```python
from build123d import *

# Parameters (mm, degrees)
SKETCH2_W           = 50.8
SKETCH2_H           = 12.7
BOSS_EXTRUDE1_DEPTH = 88.9
FILLET2_R           = 3.175
SHELL1_T            = 6.35


with BuildPart() as part:
    # Sketch2 → Boss-Extrude1 (new body)
    with BuildSketch(Plane(origin=(0, 0, 0), x_dir=(1, 0, 0), z_dir=(0, 1, 0))):
        with Locations((25.4, 6.35)):
            Rectangle(SKETCH2_W, SKETCH2_H)
    extrude(amount=BOSS_EXTRUDE1_DEPTH)

    # Fillet2
    fillet2_edges = [part.edges().sort_by_distance(p)[0] for p in [
        (50.8, 44.45, 0),
        (0, 44.45, 0),
    ]]
    fillet(fillet2_edges, radius=FILLET2_R)

    # Shell1
    shell1_openings = [part.faces().sort_by_distance(p)[0] for p in [
        (25.4, 0, -6.38808439),
        (25.4, 88.9, -6.38808439),
        (25.4, 44.45, -12.7),
    ]]
    offset(amount=SHELL1_T, openings=shell1_openings, kind=Kind.INTERSECTION)


solid = part.part
```
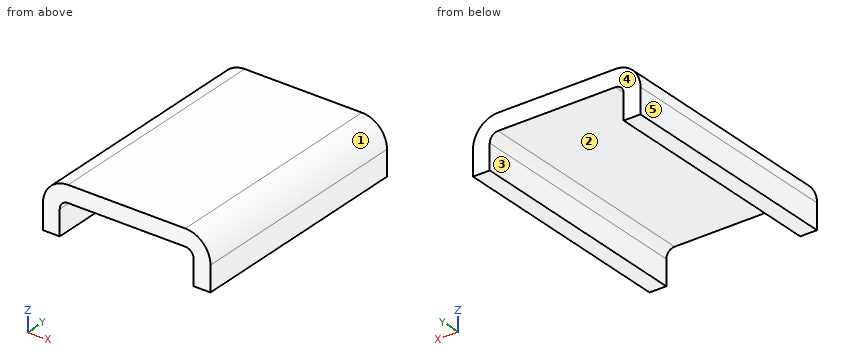
Could you check a few things on this model? Use its own coordinates, in mm. Face numbers are marked on the shaded views. A direction names the side the tool comes from. Give positions to 0.01 mm unless a question says otherwise; leave off trailing zeros. Write each loop counter-clockwise with the first axis right and the second up, starting at its lowest first coordinate (ties: lowest second). Pieces come first, ordered by that corner, then holes. Notation, with made-up numbers: (25.25, 7.25) - (77.25, 7.25) arc R23 cw to (77.25, 42.25) - close; hole circle Ø5 at (3, -15.5). An arc over 180 degrees is marked (long way). One line per item, written item: value. Start each with the question number.
Item 1: Imagine slicing it at A-A, the plane y = 62. List the corners of the cut face in (x, z) for me (3 decimals), and give its area (3 significant figures).
Item 2: Imagine slicing it at B-B, the plane z = -7.25. List the corners of the cut face in (x, y) for me.
Item 3: Imagine slicing it at C-C, the plane x = 28. List the corners of the cut face in (y, z) for me, and give its area (3 significant figures).
Item 4: I'm going to push flat-ended pins straight in: pin 1 (1.5 mm diameter, centred on y = 73, z = 3.5, fed in from +X); pin 2 (10 mm diameter, centred on y = 38.5, z = 1.5, fed in from +X); pin 3 (5 mm diameter, centred on x = 34.5, y = 69.5, fed in from -Z). Where does each tip first touch, or does it pass through?
Item 5: Which directions (+Z, -Z, +X, -X, +Y, -Y) give clear straight access to the entire face, cutting with the end or side of a thin tool? Please do the marked faces 1 and 2.
Item 6: Imagine slicing it at D-D, the plane z = 2. List the corners of the cut face in (x, y) for me.
Item 7: If we mould it in two halves opening along X, with no side actions, what happens to the marked faces 3, 4 and 5? For each: +X half, -X half, draft (parallel to the pull), parting line (faces both ways), or undercut.
Item 8: Please list where these lines run through material, in increasing order: line 1 (X direction, y = 79, z = -11.5); line 2 (Z direction, x = 25, y = 46). Write a range as from..to.
Geometry says:
1. outline: (-6.35, -12.7) - (0, -12.7) - (0, -3.175) arc R3.175 cw to (3.175, 0) - (47.625, 0) arc R3.175 cw to (50.8, -3.175) - (50.8, -12.7) - (57.15, -12.7) - (57.15, -3.175) arc R9.525 ccw to (47.625, 6.35) - (3.175, 6.35) arc R9.525 ccw to (-6.35, -3.175) - close
1. area: 530 mm^2
2. outline: (-6.35, 0) - (0, 0) - (0, 88.9) - (-6.35, 88.9) - close; (50.8, 0) - (57.15, 0) - (57.15, 88.9) - (50.8, 88.9) - close
3. outline: (0, 0) - (88.9, 0) - (88.9, 6.35) - (0, 6.35) - close
3. area: 565 mm^2
4. pin 1: x = 55.08
4. pin 2: x = 57.15
4. pin 3: z = 0
5. face 1: +Z, +X, +Y, -Y
5. face 2: -Z, +Y, -Y
6. outline: (-4.82, 0) - (55.62, 0) - (55.62, 88.9) - (-4.82, 88.9) - close
7. face 3: undercut
7. face 4: draft
7. face 5: -X half
8. line 1: -6.35..0, 50.8..57.15
8. line 2: 0..6.35
